```python
from build123d import *

# Parameters (mm, degrees)
F0_W     = 1168.4
F0_H     = 609.6
F1_DEPTH = 685.8
F1_TAPER = 5
F2_T     = -12.7


with BuildPart() as f1:
    # F0 (on Top) → F1 (new body)
    with BuildSketch(Plane.XY):
        Rectangle(F0_W, F0_H)
    extrude(amount=F1_DEPTH, taper=F1_TAPER)

    # F2
    f2_openings = [f1.faces().sort_by_distance(p)[0] for p in [
        (0, 0, 0),
    ]]
    offset(amount=F2_T, openings=f2_openings)


solid = f1.part
```
Check sheet for the modelled part. Datum: model origin and axes. Units: mm. A direction names the side the tool comes from. Give positions to 0.01 mm unless a question says otherwise; leave off trailing zeros. Loops run counter-clockwise (first coordinate to the right, second up) from the corner with the lowest first, then second, coordinate; pieces in that order, holes last. Notation, with made-up numbers: M 52,30.5 L 89,30.5 A21 cw 89,55.5 Z; hole C -17,58 d1. An arc over 180 degrees is marked long. Answer as CSV lines item,"result".
Item 1: Sectioned sample at C-C, the plane z = 83.5. Enter the section's corners in (x, y), then the cut area to 3 significant figures.
Reply:
outline,"M -576.89,-297.49 L 576.89,-297.49 L 576.89,297.49 L -576.89,297.49 Z; hole M -564.15,-284.75 L 564.15,-284.75 L 564.15,284.75 L -564.15,284.75 Z"
area,"43,900 mm^2"
Item 2: Depth check by flat-ended pin: pin 1 Ø4 at (y, z) = (-90, 232) entering from -X; pin 2 Ø1.5 at (x, z) = (-208.5, 299.5) entering from -Y; pin 3 Ø8 at (y, z) = (241.5, 523.5) entering from -X. Enter the tip coordinate at first touch or a pass-through.
Reply:
pin 1,"x = -564.08"
pin 2,"y = -278.66"
pin 3,"x = -538.75"
Item 3: Sectioned sample at B-B, the plane x = -380.5. Enter the section's corners in (y, z), then the cut area to 3 significant figures.
Reply:
outline,"M -304.8,0 L -292.05,0 L -233.16,673.1 L 233.16,673.1 L 292.05,0 L 304.8,0 L 244.8,685.8 L -244.8,685.8 Z"
area,"23,400 mm^2"
Item 4: Set-up check for faces 1 (the face through (8.18, -275.22, 338.1)), 2 (the face through (542.42, 4.09, 331.84)): record each of +Z, -Z, +X, -X, +Y, -Y from which the full face is reachable in a straight line by a thin tool's end or side.
Reply:
face 1,"+Z, +X, -X, -Y"
face 2,"-Z"
Item 5: Sectioned sample at D-D, the plane z = 452. Enter the section's corners in (x, y).
Reply:
outline,"M -544.66,-265.26 L 544.66,-265.26 L 544.66,265.26 L -544.66,265.26 Z; hole M -531.91,-252.51 L 531.91,-252.51 L 531.91,252.51 L -531.91,252.51 Z"
Item 6: Draft check along X on faces 3 (the face through (554.62, 4.27, 338.1)), 4 (the face through (8, -263.02, 331.84)), 5 (the face through (-554.62, -4.27, 338.1)), 6 (the face through (-8.18, 275.22, 338.1)). Enter one of: pulls with the +X half, pulls with the -X half, needs draft (parallel to the pull), parting line crosses it, or undercut.
Reply:
face 3,"pulls with the +X half"
face 4,"undercut"
face 5,"pulls with the -X half"
face 6,"needs draft"
Item 7: Scan lines: L1, parallel to Z at x = 201.5, y = 101; L2, parallel to X at y = -76.5, z = 314; L3, parallel to Y at x = 486, z = 201.5. Record each from-to range of solid material in increasing order.
Reply:
L1,"673.1 to 685.8"
L2,"-556.73 to -543.98, 543.98 to 556.73"
L3,"-287.17 to -274.42, 274.42 to 287.17"
Item 8: Sectioned sample at A-A, the plane y = -8. Enter the section's corners in (x, z), then the cut area to 3 significant figures.
Reply:
outline,"M -584.2,0 L -571.45,0 L -512.56,673.1 L 512.56,673.1 L 571.45,0 L 584.2,0 L 524.2,685.8 L -524.2,685.8 Z"
area,"30,500 mm^2"
